The drawing under review shows one solid part. Ordinate dimensions are in mm from its lowest x, y, z. A direction names the side the tool comes from. Round coordinates to 2 decimals unless told otherwise and drop trailing zeros. Write each loop counter-clockwise with the first axis right and the second up, starting at its lowest first coordinate (ties: lowest second). Pieces come first, ordered by that corner, then holes. Notation, with made-up numbers: (75.5, 85.5) -> (87.5, 85.5) arc R18 ccw to (87.5, 120.5) -> close; hole circle Ø2 at (62, -19). An arc over 180 degrees is marked (long way). Answer in a Markdown table with one row per item.
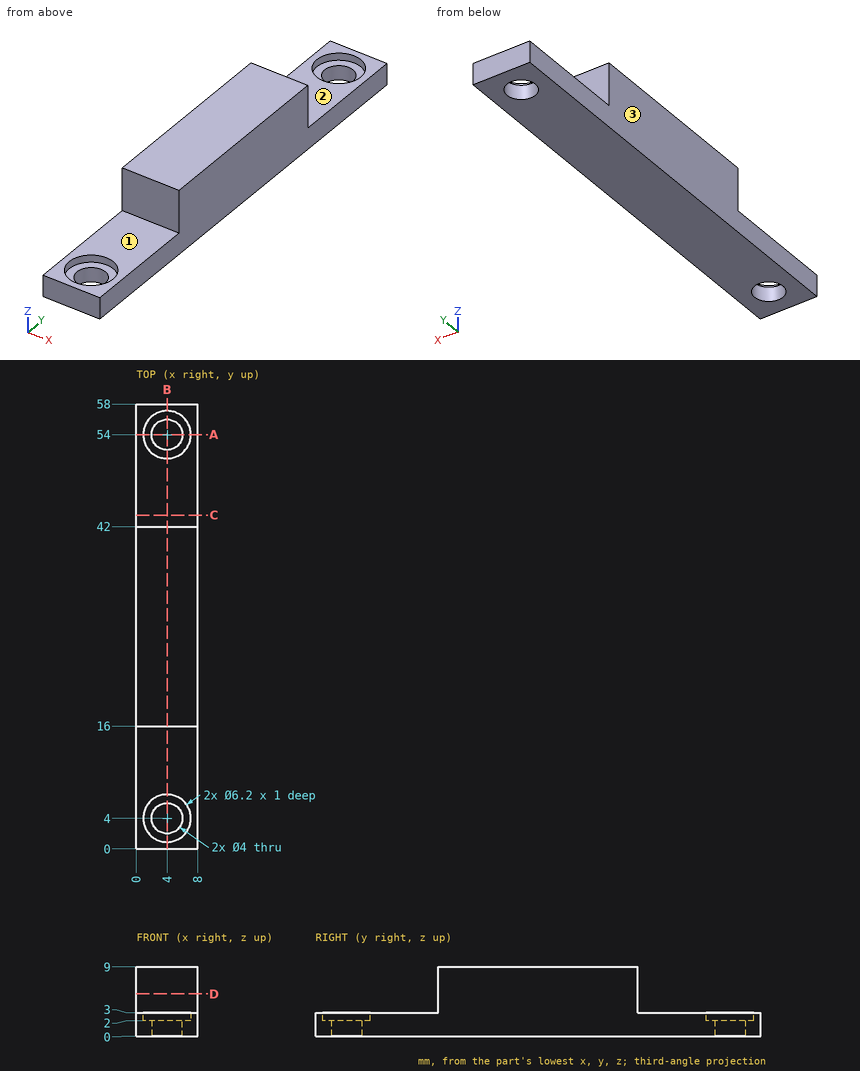
1) For the marked faces 1, 2 and 3, list the 3-axis set-ups (+Z, -Z, +X, -X, +Y, -Y) from which the entire face can be reached by the end or side of a thin tool; tool diameter is ignored.
Solved:
| item | result |
|---|---|
| face 1 | +Z, +X, -X, -Y |
| face 2 | +Z, +X, -X, +Y |
| face 3 | +Z, -Z, -X, +Y, -Y |
2) Consider section C-C on y = 43.5. State the section outline as (x, z) points, then the cut area to 3 significant figures.
Solved:
| item | result |
|---|---|
| outline | (0, 0) -> (8, 0) -> (8, 3) -> (0, 3) -> close |
| area | 24.0 mm² |
3) Consider section A-A on y = 54. State the section outline as (x, z) points, then the cut area to 3 significant figures.
Solved:
| item | result |
|---|---|
| outline | (0, 0) -> (2, 0) -> (2, 2) -> (0.9, 2) -> (0.9, 3) -> (0, 3) -> close; (6, 0) -> (8, 0) -> (8, 3) -> (7.1, 3) -> (7.1, 2) -> (6, 2) -> close |
| area | 9.80 mm² |
4) For line 1 (Y direction, x = 4, z = 0.95); line 2 (Y direction, x = 4, z = 2.2); line 3 (X direction, y = 4, z = 0.85), list the stretches that pass through material, from the lowest coordinate up. Write a range as [from, to].
Solved:
| item | result |
|---|---|
| line 1 | [0, 2], [6, 52], [56, 58] |
| line 2 | [0, 0.9], [7.1, 50.9], [57.1, 58] |
| line 3 | [0, 2], [6, 8] |
5) Consider section B-B on x = 4. State the section outline as (y, z) points, then the cut area to 3 significant figures.
Solved:
| item | result |
|---|---|
| outline | (0, 0) -> (2, 0) -> (2, 2) -> (0.9, 2) -> (0.9, 3) -> (0, 3) -> close; (6, 0) -> (52, 0) -> (52, 2) -> (50.9, 2) -> (50.9, 3) -> (42, 3) -> (42, 9) -> (16, 9) -> (16, 3) -> (7.1, 3) -> (7.1, 2) -> (6, 2) -> close; (56, 0) -> (58, 0) -> (58, 3) -> (57.1, 3) -> (57.1, 2) -> (56, 2) -> close |
| area | 302 mm² |
6) Clearance check with flat-ended pins moving along their axes: pin 1 Ø2 at (x, y) = (7, 48.5) entering from -Z; pin 2 Ø4.5 at (x, y) = (4, 54) entering from +Z; pin 3 Ø2.5 at (x, y) = (5.5, 7) entering from +Z. State where each tip first meets the part, or that it passes through.
Solved:
| item | result |
|---|---|
| pin 1 | z = 0 |
| pin 2 | z = 2 |
| pin 3 | z = 3 |
7) Consider section D-D on z = 5.5. State the section outline as (x, y) points, then the cut area to 3 significant figures.
Solved:
| item | result |
|---|---|
| outline | (0, 16) -> (8, 16) -> (8, 42) -> (0, 42) -> close |
| area | 208 mm² |
